The listing builds one solid part. Answer for the finished solid, in the listing's coordinates (mm). A direction names the side the tool comes from. Coordinates: 2 decimals unless noted, no trailing zeros. Order: outer loops, then holes, each group sorted by start corner. A loop starts at its lowest first (then second) coordinate and runs counter-clockwise, first axis right, second up. Notation, with made-up numbers: (27.25, 78) -> (74.25, 78) arc R17 cw to (74.25, 85) -> close; hole circle Ø9 at (63, 76). An arc over 180 degrees is marked (long way). Write item = value, one per line.
from build123d import *

# Parameters (mm, degrees)
SKETCH1_R           = 7.5
BOSS_EXTRUDE3_DEPTH = 10
SKETCH54_R          = 10.540559159
BOSS_EXTRUDE5_DEPTH = 3.040559
BOSS_EXTRUDE5_TAPER = 45
SKETCH55_R          = 10.540559159
BOSS_EXTRUDE6_DEPTH = 3.040559
BOSS_EXTRUDE6_TAPER = 45
SKETCH56_R          = 10.540559159
BOSS_EXTRUDE7_DEPTH = 3.918882
SKETCH53_R          = 6.5
CUT_EXTRUDE7_DEPTH  = 11.0000001
SKETCH57_R          = 7.5
SKETCH57_R_2        = 6.5
CUT_EXTRUDE8_DEPTH  = 1
SKETCH59_R          = 7.5
SKETCH59_R_2        = 6.5
CUT_EXTRUDE9_DEPTH  = 1


with BuildPart() as part:
    # Sketch1 → Boss-Extrude3 (new body)
    with BuildSketch(Plane(origin=(0, 0, 0), x_dir=(1, 0, 0), z_dir=(0, 1, 0))):
        Circle(SKETCH1_R)
    extrude(amount=BOSS_EXTRUDE3_DEPTH)

    # Sketch54 → Boss-Extrude5 (add)
    with BuildSketch(Plane(origin=(0, 6.959440841, 0), x_dir=(1, 0, 0), z_dir=(0, 1, 0))):
        Circle(SKETCH54_R)
    extrude(amount=BOSS_EXTRUDE5_DEPTH, taper=BOSS_EXTRUDE5_TAPER)

    # Sketch55 → Boss-Extrude6 (add)
    with BuildSketch(Plane.XZ.offset(-3.040559159)):
        Circle(SKETCH55_R)
    extrude(amount=BOSS_EXTRUDE6_DEPTH, taper=BOSS_EXTRUDE6_TAPER)

    # Sketch56 → Boss-Extrude7 (add)
    with BuildSketch(Plane(origin=(0, 6.959440841, 0), x_dir=(-1, 0, 0), z_dir=(0, -1, 0))):
        Circle(SKETCH56_R)
    extrude(amount=BOSS_EXTRUDE7_DEPTH)

    # Sketch53 → Cut-Extrude7 (cut, through all)
    with BuildSketch(Plane(origin=(0, 10, 0), x_dir=(1, 0, 0), z_dir=(0, 1, 0))):
        Circle(SKETCH53_R)
    extrude(amount=-CUT_EXTRUDE7_DEPTH, mode=Mode.SUBTRACT)

    # Sketch57 → Cut-Extrude8 (cut)
    with BuildSketch(Plane(origin=(0, 0, 0), x_dir=(-1, 0, 0), z_dir=(0, -1, 0))):
        Circle(SKETCH57_R)
        Circle(SKETCH57_R_2, mode=Mode.SUBTRACT)
    extrude(amount=-CUT_EXTRUDE8_DEPTH, mode=Mode.SUBTRACT)

    # Sketch59 → Cut-Extrude9 (cut)
    with BuildSketch(Plane(origin=(0, 10, 0), x_dir=(1, 0, 0), z_dir=(0, 1, 0))):
        Circle(SKETCH59_R)
        Circle(SKETCH59_R_2, mode=Mode.SUBTRACT)
    extrude(amount=-CUT_EXTRUDE9_DEPTH, mode=Mode.SUBTRACT)


solid = part.part
Q1. Section B-B, the plane y = 5.5 is taken. Give the vertices of the cut face in (x, z).
The answers:
outline = circle Ø21.08 at (0, 0); hole circle Ø13 at (0, 0)
Q2. Find the intervals of material crossed by line 1 along X through (y, z) = (4.5, 0); line 2 along X through (y, z) = (8, 2.75); line 3 along Z through (x, y) = (-3.75, 5), in increasing order.
The answers:
line_1 = -10.54 to -6.5, 6.5 to 10.54
line_2 = -9.09 to -5.89, 5.89 to 9.09
line_3 = -9.85 to -5.31, 5.31 to 9.85
Q3. A tool of negligible diameter and unlimited length cuts with its end or side. For faces 1 (the face through (2.28, 5.03, 10.29)), 2 (the face through (-7.493, 9.507, -0.33)), 3 (the face through (6, 1, -3)), from which of +Z, -Z, +X, -X, +Y, -Y can it reach the whole face along a straight path? Write none if from no direction.
The answers:
face_1 = +Y, -Y
face_2 = +Y
face_3 = -Y
Q4. Each of these flat-tipped pins is pushed along its axis until it touches: pin 1 Ø5 at (y, z) = (3.5, 7) entering from -X; pin 2 Ø6 at (y, z) = (7.5, -4) entering from -X; pin 3 Ø4.5 at (x, z) = (0.5, -3.5) entering from -Y; pin 4 Ø1 at (y, z) = (3, 6) entering from +X. Where does it stop, or does it pass through?
The answers:
pin_1 = -9.53
pin_2 = -10.49
pin_3 = through
pin_4 = 8.99
Q5. Section A-A, the plane x = 0 is taken. Give the vertices of the cut face in (y, z), plus the area to 3 significant figures.
The answers:
outline = (0, -7.5) -> (3.04, -10.54) -> (6.96, -10.54) -> (10, -7.5) -> (9, -7.5) -> (9, -6.5) -> (1, -6.5) -> (1, -7.5) -> close; (0, 7.5) -> (1, 7.5) -> (1, 6.5) -> (9, 6.5) -> (9, 7.5) -> (10, 7.5) -> (6.96, 10.54) -> (3.04, 10.54) -> close
area = 58.3 mm2
Q6. The mould has two halves that part along Z. Classify faces 4 (the face through (-1.66, 0.15, -7.47)), 5 (the face through (7.493, 0.493, -0.33)): released by +Z, released by -Z, zero draft, split by the parting line, or undercut.
The answers:
face_4 = split by the parting line
face_5 = undercut
